```python
from build123d import *

# Parameters (mm, degrees)
BOSS_EXTRU_1_DEPTH      = 10
ESQUISSE2_R             = 1.5
ENL_V_MAT_EXTRU_1_DEPTH = 20


with BuildPart() as part:
    # Esquisse1 → Boss.-Extru.1 (new body)
    with BuildSketch(Plane.XY):
        with BuildLine():
            Line((0, 1.373626374), (0, 11.373626374))
            Line((0, 11.373626374), (12, 11.373626374))
            Line((12, 11.373626374), (12, 1.373626374))
            Line((12, 1.373626374), (22, 1.373626374))
            Line((22, 1.373626374), (22, 6.373626374))
            Line((22, 6.373626374), (17, 6.373626374))
            Line((17, 6.373626374), (17, 13.373626374))
            ThreePointArc((17, 13.373626374), (16.121320344, 15.494946717), (14, 16.373626374))
            Line((14, 16.373626374), (-2, 16.373626374))
            ThreePointArc((-2, 16.373626374), (-4.121320344, 15.494946717), (-5, 13.373626374))
            Line((-5, 13.373626374), (-5, 6.373626374))
            Line((-5, 6.373626374), (-10, 6.373626374))
            Line((-10, 6.373626374), (-10, 1.373626374))
            Line((-10, 1.373626374), (0, 1.373626374))
        make_face()
    extrude(amount=BOSS_EXTRU_1_DEPTH)

    # Esquisse2 → Enlèv. mat.-Extru.1 (cut)
    with BuildSketch(Plane(origin=(0, 6.373626374, 0), x_dir=(1, 0, 0), z_dir=(0, 1, 0))):
        with Locations((-7.5, -15)):
            Circle(ESQUISSE2_R)
        with Locations(Location((-7.5, -5, 0), (0, 0, 270))):
            Circle(ESQUISSE2_R)
        with Locations(Location((19.5, -5, 0), (0, 0, 270))):
            Circle(ESQUISSE2_R)
        with Locations((19.5, -15)):
            Circle(ESQUISSE2_R)
    extrude(amount=-ENL_V_MAT_EXTRU_1_DEPTH, mode=Mode.SUBTRACT)


solid = part.part
```
Read the model definition and answer for the solid it produces. Units are mm, in the model's axes. A direction names the side the tool comes from. Give positions to 0.01 mm unless a question says otherwise; leave off trailing zeros. Order: outer loops, then holes, each group sorted by start corner. A loop starts at its lowest first (then second) coordinate and runs counter-clockwise, first axis right, second up. Notation, with made-up numbers: (-22.5, 55.5) -> (34.5, 55.5) arc R27 ccw to (34.5, 76.5) -> close; hole circle Ø10 at (88, 50.25). An arc over 180 degrees is marked (long way). One line per item, written item: value. Start each with the question number.
(1) The part is cut by section A-A (z = 5). Determine the outline of the cut face in (x, y), and give its area (3 significant figures).
(2) For a pull along X with two mould halves and no side action, classify faces 6 (the flat face through (6, 16.374, 5)), 7 (the flat face through (12, 6, 5)), 8 (the cylindrical face through (20.765, 3.909, 5.806)), 9 (the flat face through (-10, 4, 5)) as released by +X, released by -X, zero draft, split by the parting line, or undercut.
(3) A tool of negligible diameter and unlimited length cuts with its end or side. For faces 1 (the flat face through (22, 4, 5)), 2 (the flat face through (6, 12, 10)), 3 (the flat face through (21, 6.374, 4)), 4 (the flat face through (6, 11.374, 5)), 5 (the flat face through (-6, 6.374, 4)), from which of +Z, -Z, +X, -X, +Y, -Y can it reach the whole face along a straight path? Write none if from no direction.
(4) The part is cut by section D-D (y = 10.25). Determine the outline of the cut face in (x, z), and give its area (3 significant figures).
(5) The part is cut by section B-B (y = 5). Determine the outline of the cut face in (x, z), and give its area (3 significant figures).
(6) Flat-ended cylindrical pins translate along their axes: P1, Ø4, axis at x = -7.5, z = 5, coming from the +Y side; P2, Ø3.5, axis at y = 10.5, z = 4, coming from the -X side; P3, Ø1.5, axis at x = 9, z = 5.5, coming from the -Y side. Find the tip coordinate at first contact, or state that the pin passes through.
(7) The part is cut by section C-C (x = -7.5). Determine the outline of the cut face in (y, z), and give its area (3 significant figures).
(8) Straight lines are drawn through the part: L1, parallel to X at y = 4.8, z = 5; L2, parallel to X at y = 8.25, z = 8.5; L3, parallel to Y at x = 4, z = 5.5. For each, find the intervals that lie inside material, in ascending order.
Taken from the geometry:
1. outline: (-10, 1.37) -> (-9, 1.37) -> (-9, 6.37) -> (-10, 6.37) -> close; (-6, 1.37) -> (0, 1.37) -> (0, 11.37) -> (12, 11.37) -> (12, 1.37) -> (18, 1.37) -> (18, 6.37) -> (17, 6.37) -> (17, 13.37) arc R3 ccw to (14, 16.37) -> (-2, 16.37) arc R3 ccw to (-5, 13.37) -> (-5, 6.37) -> (-6, 6.37) -> close; (21, 1.37) -> (22, 1.37) -> (22, 6.37) -> (21, 6.37) -> close
1. area: 226 mm^2
2. face 6: zero draft
2. face 7: undercut
2. face 8: undercut
2. face 9: released by -X
3. face 1: +Z, -Z, +X, +Y, -Y
3. face 2: +Z, +X, -X, +Y, -Y
3. face 3: +Z, -Z, +X, +Y
3. face 4: +Z, -Z, -Y
3. face 5: +Z, -Z, -X, +Y
4. outline: (-5, 0) -> (0, 0) -> (0, 10) -> (-5, 10) -> close; (12, 0) -> (17, 0) -> (17, 10) -> (12, 10) -> close
4. area: 100 mm^2
5. outline: (-10, 0) -> (0, 0) -> (0, 10) -> (-10, 10) -> close; (12, 0) -> (22, 0) -> (22, 10) -> (12, 10) -> close; hole circle Ø3 at (-7.5, 5); hole circle Ø3 at (19.5, 5)
5. area: 186 mm^2
6. P1: y = 6.37
6. P2: x = -5
6. P3: y = 11.37
7. outline: (1.37, 0) -> (6.37, 0) -> (6.37, 3.5) -> (1.37, 3.5) -> close; (1.37, 6.5) -> (6.37, 6.5) -> (6.37, 10) -> (1.37, 10) -> close
7. area: 35.0 mm^2
8. L1: -10 to -9, -6 to 0, 12 to 18, 21 to 22
8. L2: -5 to 0, 12 to 17
8. L3: 11.37 to 16.37
